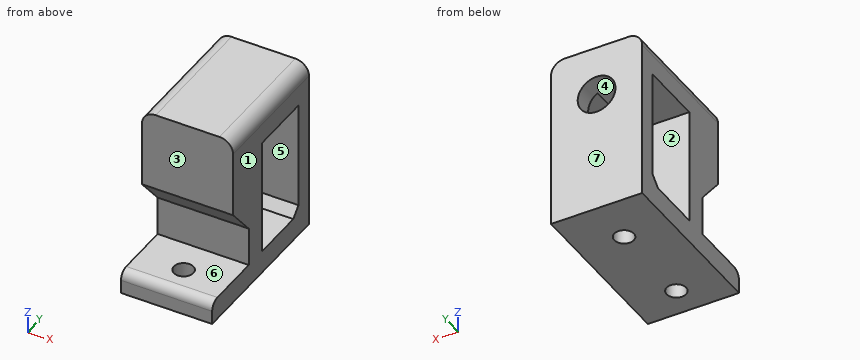
```python
from build123d import *

# Parameters (mm, degrees)
SKETCH1_W           = 20
SKETCH1_H           = 33
SKETCH1_R           = 2.15
BOSS_EXTRUDE1_DEPTH = 5
SKETCH2_W           = 20
SKETCH2_H           = 4
BOSS_EXTRUDE2_DEPTH = 38
SKETCH4_W           = 20
SKETCH4_H           = 7.411842069
BOSS_EXTRUDE3_DEPTH = 25
FILLET1_R           = 3
FILLET2_R           = 2
CHAMFER2_SIZE       = 2
SKETCH8_W           = 20
SKETCH8_H           = 5
BOSS_EXTRUDE5_DEPTH = 25.588158
SKETCH12_W          = 20
SKETCH12_H          = 10
BOSS_EXTRUDE6_DEPTH = 14
SKETCH3_R           = 4.15
CUT_EXTRUDE2_DEPTH  = 18
SKETCH15_W          = 20
SKETCH15_H          = 6
BOSS_EXTRUDE7_DEPTH = 10
SKETCH16_W          = 20
SKETCH16_H          = 14
CUT_EXTRUDE4_DEPTH  = 10
BOSS_EXTRUDE8_DEPTH = 20


with BuildPart() as part:
    # Sketch1 → Boss-Extrude1 (new body)
    with BuildSketch(Plane.XY):
        with Locations((10, -16.5)):
            Rectangle(SKETCH1_W, SKETCH1_H)
        with Locations((10, -6.5)):
            Circle(SKETCH1_R, mode=Mode.SUBTRACT)
        with Locations((10, -26.5)):
            Circle(SKETCH1_R, mode=Mode.SUBTRACT)
    extrude(amount=BOSS_EXTRUDE1_DEPTH)

    # Sketch2 → Boss-Extrude2 (add)
    with BuildSketch(Plane(origin=(0, 0, 0), x_dir=(-1, 0, 0), z_dir=(0, 0, -1))):
        with Locations((-10, 2)):
            Rectangle(SKETCH2_W, SKETCH2_H)
    extrude(amount=-BOSS_EXTRUDE2_DEPTH)

    # Sketch4 → Boss-Extrude3 (add)
    with BuildSketch(Plane.XZ):
        with Locations((10, 34.294078965)):
            Rectangle(SKETCH4_W, SKETCH4_H)
    extrude(amount=BOSS_EXTRUDE3_DEPTH)

    # Fillet1
    fillet1_edges = [part.edges().sort_by_distance(p)[0] for p in [
        (20, -10.5, 38),
        (0, -10.5, 38),
    ]]
    fillet(fillet1_edges, radius=FILLET1_R)

    # Fillet2
    fillet2_edges = [part.edges().sort_by_distance(p)[0] for p in [
        (10, -33, 5),
    ]]
    fillet(fillet2_edges, radius=FILLET2_R)

    # Chamfer2
    chamfer2_edges = [part.edges().sort_by_distance(p)[0] for p in [
        (10, 0, 5),
    ]]
    chamfer(chamfer2_edges, length=CHAMFER2_SIZE)

    # Sketch8 → Boss-Extrude5 (add)
    with BuildSketch(Plane.XY.offset(5)):
        with Locations((10, -16.5)):
            Rectangle(SKETCH8_W, SKETCH8_H)
    extrude(amount=BOSS_EXTRUDE5_DEPTH)

    # Sketch12 → Boss-Extrude6 (add)
    with BuildSketch(Plane(origin=(0, -14, 0), x_dir=(1, 0, 0), z_dir=(0, 1, 0))):
        with Locations((10, -25.588157931)):
            Rectangle(SKETCH12_W, SKETCH12_H)
    extrude(amount=BOSS_EXTRUDE6_DEPTH)

    # Sketch3 → Cut-Extrude2 (cut)
    with BuildSketch(Plane(origin=(0, 4, 0), x_dir=(1, 0, 0), z_dir=(0, 1, 0))):
        with Locations((10, -27)):
            Circle(SKETCH3_R)
    extrude(amount=-CUT_EXTRUDE2_DEPTH, mode=Mode.SUBTRACT)

    # Sketch15 → Boss-Extrude7 (add)
    with BuildSketch(Plane(origin=(0, 0, 30.588157931), x_dir=(-1, 0, 0), z_dir=(0, 0, -1))):
        with Locations((-10, -22)):
            Rectangle(SKETCH15_W, SKETCH15_H)
    extrude(amount=BOSS_EXTRUDE7_DEPTH)

    # Sketch16 → Cut-Extrude4 (cut)
    with BuildSketch(Plane(origin=(0, 0, 20.588157931), x_dir=(-1, 0, 0), z_dir=(0, 0, -1))):
        with Locations((-10, -7)):
            Rectangle(SKETCH16_W, SKETCH16_H)
    extrude(amount=-CUT_EXTRUDE4_DEPTH, mode=Mode.SUBTRACT)

    # Sketch17 → Boss-Extrude8 (add)
    with BuildSketch(Plane(origin=(20, 0, 0), x_dir=(0, 0, -1), z_dir=(1, 0, 0))):
        Polygon((-20.588157931, -19), (-20.588157931, -25), (-13.588157931, -19), align=None)
    extrude(amount=-BOSS_EXTRUDE8_DEPTH)


solid = part.part
```
Geometry check sheet. Reference: the model listing, model coordinates, mm. Face numbers are marked on the shaded views. A direction names the side the tool comes from. Give positions to 0.01 mm unless a question says otherwise; leave off trailing zeros. Loops run counter-clockwise (first coordinate to the right, second up) from the corner with the lowest first, then second, coordinate; pieces in that order, holes last. Notation, with made-up numbers: M 30,41.25 L 45,41.25 A32 cw 45,68.25 Z; hole C -31.5,32 d10. An arc over 180 degrees is marked long. Write item = value, one per line. Start each with the question number.
1. Section check B-B, the plane z = 27. Enter the section's corners in (x, y), plus the area to 3 significant figures.
2. Section check C-C, the plane x = 10. Enter the section's corners in (y, z).
3. Thickness scan on probe 1 along Y at (x, z) = (10, 2.8); probe 2 along Z at (x, y) = (7.5, -4.5); probe 3 along Y at (x, z) = (17.5, 29). Record the ranges inside material, lowest first.
4. Section check A-A, the plane y = -26.5. Enter the section's corners in (x, z).
5. Tool access check on the marked faces 4, 5, 6 and 7. Record the directions out of +Z, -Z, +X, -X, +Y, -Y that give a thin tool (end or side, any length) a straight path to the whole face; none if there is none.
6. Draft check along Y on the marked faces 1, 2 and 3. Enter one of: +Y half, -Y half, draft (parallel to the pull), parting line (faces both ways), or undercut.
7. Section check D-D, the plane y = -6.5. Enter the section's corners in (x, z).
8. Go/stop test with flat-tipped pins: P1, Ø10, axis at x = 9.5, z = 21.5, coming from the -Y side; P2, Ø1, axis at x = 9, z = 8.5, coming from the -Y side; P3, Ø3, axis at x = 12.5, y = -2.5, coming from the -Z side; P4, Ø8, axis at x = 5.5, z = 16.5, coming from the -Y side. Record where each tip stops, or that it passes through.
Values follow:
q1.outline = M 0,-25 L 20,-25 L 20,-14 L 0,-14 Z; M 0,0 L 5.85,0 L 5.85,4 L 0,4 Z; M 14.15,0 L 20,0 L 20,4 L 14.15,4 Z
q1.area = 267 mm^2
q2.outline = M -33,0 L -28.65,0 L -28.65,5 L -31,5 A2 ccw -33,3 Z; M -25,20.59 L -19,13.59 L -19,5 L -24.35,5 L -24.35,0 L -8.65,0 L -8.65,5 L -14,5 L -14,31.15 L 4,31.15 L 4,38 L -25,38 Z; M -4.35,0 L 4,0 L 4,22.85 L 0,22.85 L 0,7 L -2,5 L -4.35,5 Z
q3.probe_1 = -33 to -28.65, -24.35 to -8.65, -4.35 to 4
q3.probe_2 = 0 to 5, 30.59 to 38
q3.probe_3 = -25 to -14, 0 to 4
q4.outline = M 0,0 L 7.85,0 L 7.85,5 L 0,5 Z; M 12.15,0 L 20,0 L 20,5 L 12.15,5 Z
q5.face_4 = +Y
q5.face_5 = +X, -X
q5.face_6 = +X, -X, -Y
q5.face_7 = +Z, -Z, +X, -X, +Y
q6.face_1 = draft
q6.face_2 = undercut
q6.face_3 = -Y half
q7.outline = M 0,0 L 7.85,0 L 7.85,5 L 0,5 Z; M 0,30.59 L 7.91,30.59 A4.15 cw 12.09,30.59 L 20,30.59 L 20,35 A3 ccw 17,38 L 3,38 A3 ccw 0,35 Z; M 12.15,0 L 20,0 L 20,5 L 12.15,5 Z
q8.P1 = -25
q8.P2 = -19
q8.P3 = 0
q8.P4 = -24.92
